Model file for the job. Use its own axes, mm. Face numbers are marked on the shaded views. Round coordinates to 2 decimals unless told otherwise and drop trailing zeros. Order: outer loops, then holes, each group sorted by start corner. A loop starts at its lowest first (then second) coordinate and runs counter-clockwise, first axis right, second up. Notation, with made-up numbers: (89.5, -34) -> (114.5, -34) arc R21 ccw to (114.5, -25) -> close; hole circle Ø10 at (64, -28). An arc over 180 degrees is marked (long way). Put each result on its own line as item: value. Start each with the question number.
Q1. Pull direction X, two halves, no side cores. Call the marked faces 1, 2 and 3: released by +X, released by -X, zero draft, split by the parting line, or undercut.
Q2. Flat gauge pins, fed straight in: P1, Ø2.5, axis at x = 15.5, y = -4.5, coming from the -Z side; P2, Ø1, axis at x = 5, y = -1.5, coming from the +Z side. Where does each tip first touch, or does it go through?
Q3. Probe L1, parallel to Y at x = 8, z = 0.6; L2, parallel to Z at x = 36, y = -4.5; L3, parallel to Z at x = 41, y = -2. List the from-to ranges inside material, lowest first.
Q4. Cut at B-B, the plane y = -1. List the corners of the cut face in (x, z).
Q5. Cut at A-A, the plane x = 8. List the corners of the cut face in (y, z), and give its area (3 significant figures).
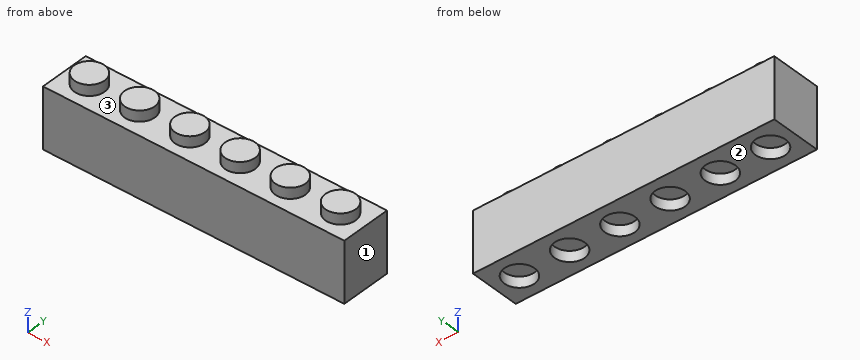
from build123d import *

# Parameters (mm, degrees)
F1_DEPTH  = 8
F3_W      = 8
F3_H      = 8
F3_R      = 2.4
F4_DEPTH  = 1.7
F5_R      = 2.4
F6_DEPTH  = 1.7
F13_W     = 22.9428485036
F13_H     = 31.0530802235
F14_DEPTH = 16.002


with BuildPart() as f1:
    # F0 (on Front) → F1 (new body)
    with BuildSketch(Plane.XZ):
        Polygon((-2.4, 9.6), (-4, 9.6), (-4, 0), (4, 0), (4, 9.6), (2.4, 9.6), (2.4, 11.3), (-2.4, 11.3), align=None)
    extrude(amount=F1_DEPTH)

    # F3 (on plane+point) → F4 (cut, through all)
    with BuildSketch(Plane.XY.offset(11.3)):
        with Locations((0, -4)):
            Rectangle(F3_W, F3_H)
        with Locations((0, -4)):
            Circle(F3_R, mode=Mode.SUBTRACT)
    extrude(amount=-F4_DEPTH, mode=Mode.SUBTRACT)

    # F5 (on Top) → F6 (cut)
    with BuildSketch(Plane.XY):
        with Locations((0, -4)):
            Circle(F5_R)
    extrude(amount=F6_DEPTH, mode=Mode.SUBTRACT)

    # F8: F1 across plane


with BuildPart() as f1_1:
    add(f1.part)
    add(f1.part.mirror(Plane.YZ.offset(4)))

    # F10: F1 across plane


with BuildPart() as f1_2:
    add(f1_1.part)
    add(f1_1.part.mirror(Plane.YZ.offset(12)))

    # F12: F1 across plane


with BuildPart() as f1_3:
    add(f1_2.part)
    add(f1_2.part.mirror(Plane.YZ.offset(28)))

    # F13 (on face) → F14 (cut)
    with BuildSketch(Plane.YZ.offset(60)):
        with Locations((-3.3198129386, 4.1634761728)):
            Rectangle(F13_W, F13_H)
    extrude(amount=-F14_DEPTH, mode=Mode.SUBTRACT)


solid = f1_3.part
Ans:
1. face 1: released by +X
1. face 2: zero draft
1. face 3: undercut
2. P1: stops at z = 1.7
2. P2: stops at z = 9.6
3. L1: y = -8 to -6.4, -1.6 to 0
3. L2: z = 0 to 9.6
3. L3: z = 1.7 to 11.3
4. outline: (-4, 0) -> (44, 0) -> (44, 9.6) -> (-4, 9.6) -> close
5. outline: (-8, 0) -> (-6.4, 0) -> (-6.4, 1.7) -> (-1.6, 1.7) -> (-1.6, 0) -> (0, 0) -> (0, 9.6) -> (-1.6, 9.6) -> (-1.6, 11.3) -> (-6.4, 11.3) -> (-6.4, 9.6) -> (-8, 9.6) -> close
5. area: 76.8 mm^2
